from build123d import *

# Parameters (mm, degrees)
BOSS_EXTRUDE9_DEPTH = 90
SKETCH17_R          = 2.5
CUT_EXTRUDE1_DEPTH  = 5


with BuildPart() as part:
    # Sketch1 → Boss-Extrude9 (new body)
    with BuildSketch(Plane(origin=(0, 0, 0), x_dir=(1, 0, 0), z_dir=(0, 1, 0))):
        with BuildLine():
            ThreePointArc((-10, -68.271516755), (-17.330093713, -66.788231388), (-24.456600104, -64.520343391))
            Line((-24.456600104, -64.520343391), (-24.456600104, -67.187236223))
            ThreePointArc((-24.456600104, -67.187236223), (0, -71.5), (24.456600104, -67.187236223))
            Line((24.456600104, -67.187236223), (24.456600104, -64.520343391))
            ThreePointArc((24.456600104, -64.520343391), (17.330093713, -66.788231388), (10, -68.271516755))
            ThreePointArc((10, -68.271516755), (0, -69), (-10, -68.271516755))
        make_face()
    extrude(amount=BOSS_EXTRUDE9_DEPTH)

    # Sketch17 → Cut-Extrude1 (cut, symmetric)
    with BuildSketch(Plane.XY.offset(67.187236223)):
        with Locations((0, 75)):
            Circle(SKETCH17_R)
        with Locations((0, 45)):
            Circle(SKETCH17_R)
    extrude(amount=CUT_EXTRUDE1_DEPTH, both=True, mode=Mode.SUBTRACT)


solid = part.part
Source: CAD feature listing. Evaluate the final solid. Frame: model axes, mm. Round coordinates to 2 decimals unless told otherwise and drop trailing zeros. Loops run counter-clockwise (first coordinate to the right, second up) from the corner with the lowest first, then second, coordinate; pieces in that order, holes last. Notation, with made-up numbers: M 48.5,-7.5 L 79.5,-7.5 A26 cw 79.5,21.5 Z; hole C 81.5,57.5 d7. An arc over 180 degrees is marked long. Answer as CSV lines item,"result".
Q1. Cut plane C-C (y = 75). Return the cut outline in (x, z), plus the area to 3 significant figures.
Verdict:
outline,"M -24.46,64.52 A69 cw -2.5,68.95 L -2.5,71.46 A71.5 ccw -24.46,67.19 Z; M 2.5,68.95 A69 cw 24.46,64.52 L 24.46,67.19 A71.5 ccw 2.5,71.46 Z"
area,"112 mm^2"
Q2. Cut plane D-D (x = -19). Return the cut outline in (y, z).
Verdict:
outline,"M 0,66.33 L 90,66.33 L 90,68.93 L 0,68.93 Z"
Q3. Cut plane A-A (x = 0). Return the cut outline in (y, z), plus the area to 3 significant figures.
Verdict:
outline,"M 0,69 L 42.5,69 L 42.5,71.5 L 0,71.5 Z; M 47.5,69 L 72.5,69 L 72.5,71.5 L 47.5,71.5 Z; M 77.5,69 L 90,69 L 90,71.5 L 77.5,71.5 Z"
area,"200 mm^2"
Q4. Line query: line 1 along Y through (x, z) = (0, 69.8); line 2 along Z through (x, y) = (0.5, 69); line 3 along Z through (x, y) = (-8.5, 85). Output: solid intervals per line, ascending.
Verdict:
line 1,"y = 0 to 42.5, 47.5 to 72.5, 77.5 to 90"
line 2,"z = 69 to 71.5"
line 3,"z = 68.47 to 70.99"
Q5. Pull-direction query (X, two-part tool) for faces 1 (the face through (0, 0, 70)), 2 (the face through (-24.457, 44, 66)), 3 (the face through (-0.54, 72.56, 70.21)); classes: +X half, -X half, draft (parallel to the pull), parting line (faces both ways), or undercut.
Verdict:
face 1,"draft"
face 2,"-X half"
face 3,"undercut"
Q6. Cut plane B-B (z = 65.75). Return the cut outline in (x, y).
Verdict:
outline,"M -24.46,0 L -20.93,0 L -20.93,90 L -24.46,90 Z; M 20.93,0 L 24.46,0 L 24.46,90 L 20.93,90 Z"
Q7. Contact query for flat-ended pins moving along their axis: pin 1 (8 mm diameter, centred on x = -17, y = 13, fed in from -Z); pin 2 (1.5 mm diameter, centred on x = -6.5, y = 10, fed in from -Z); pin 3 (1 mm diameter, centred on x = 3, y = 63.5, fed in from -Z); pin 4 (4.5 mm diameter, centred on x = 0, y = 75, fed in from +Z) (3 decimals). Output: stop coordinate, or through.
Verdict:
pin 1,"stops at z = 65.73"
pin 2,"stops at z = 68.62"
pin 3,"stops at z = 68.91"
pin 4,"passes through"
